```python
from build123d import *

# Parameters (mm, degrees)
F1_DEPTH = 40.2336
F0_R     = 10.16
F2_DEPTH = 15.7734
F3_R     = 3.302


with BuildPart() as f1:
    # F0 (on Front) → F1 (new body)
    with BuildSketch(Plane.XZ):
        with BuildLine():
            ThreePointArc((5.543906, -28.032048), (22.07881, -18.139922), (28.575, 0))
            ThreePointArc((28.575, 0), (22.07881, 18.139922), (5.543906, 28.032048))
            ThreePointArc((5.543906, 28.032048), (-28.575, 0), (5.543906, -28.032048))
        make_face()
        with BuildLine():
            ThreePointArc((13.447765, -4.826), (-14.2875, 0), (13.447765, 4.826))
            Line((13.447765, 4.826), (18.5293, 4.826))
            Line((18.5293, 4.826), (18.5293, -4.826))
            Line((18.5293, -4.826), (13.447765, -4.826))
        make_face(mode=Mode.SUBTRACT)
    extrude(amount=F1_DEPTH)

    # F0 (on Front) → F2 (join)
    with BuildSketch(Plane.XZ):
        with BuildLine():
            ThreePointArc((5.543906, 28.032048), (22.07881, 18.139922), (28.575, 0))
            ThreePointArc((28.575, 0), (22.07881, -18.139922), (5.543906, -28.032048))
            Line((5.543906, -28.032048), (59.169933, -18.327989))
            ThreePointArc((59.169933, -18.327989), (69.171479, -11.487798), (73.025, 0))
            ThreePointArc((73.025, 0), (69.171479, 11.487798), (59.169933, 18.327989))
            Line((59.169933, 18.327989), (5.543906, 28.032048))
        make_face()
        with Locations((53.975, 0)):
            Circle(F0_R, mode=Mode.SUBTRACT)
    extrude(amount=F2_DEPTH)

    # F3
    f3_edges = [f1.edges().sort_by_distance(p)[0] for p in [
        (-5.543906, -40.2336, 28.032048),
    ]]
    fillet(f3_edges, radius=F3_R)


solid = f1.part
```
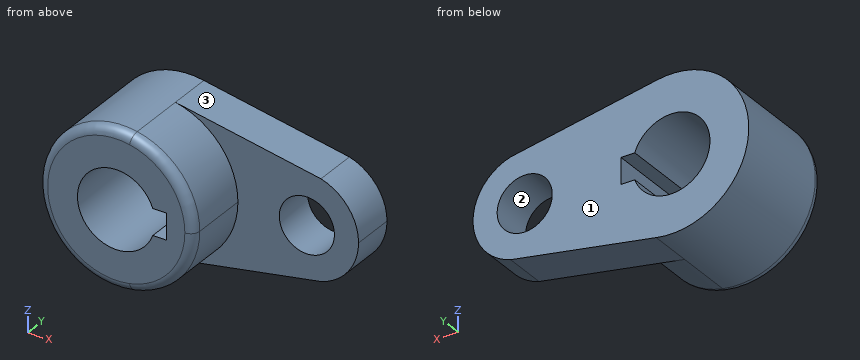
Source: CAD feature listing. Evaluate the final solid. Frame: model axes, mm. Face numbers are marked on the shaded views. Coordinates: 2 decimals unless noted, no trailing zeros. Put each result on its own line as item: value. Start each with the question number.
1) Pull-direction query (Z, two-part tool) for the marked faces 1, 2 and 3; classes: pulls with the +Z half, pulls with the -Z half, needs draft (parallel to the pull), parting line crosses it, or undercut.
2) Ray query, L1, parallel to X at y = -18.5, z = 0 (1 decimal); L2, parallel to Z at x = 0, y = -15 (1 decimal); L3, parallel to X at y = -7, z = -8.5. Return the intervals inside material, ascending. Write a range as from..to.
3) Contact query for flat-ended pins moving along their axis: pin 1 Ø5.5 at (x, y) = (17, -13) entering from -Z; pin 2 Ø4 at (x, y) = (16, -16.5) entering from +Z; pin 3 Ø8 at (x, z) = (36.5, -10.5) entering from -Y. Output: stop coordinate, or through.
4) Cut plane A-A on y = -5. Give the number of separate pieces and of enclosed holes in the cut face, then the cut area to 3 significant figures.
The answers:
1. face 1: needs draft
1. face 2: undercut
1. face 3: pulls with the +Z half
2. L1: x = -28.6..-14.3, 18.5..28.6
2. L2: z = -28.6..-14.3, 14.3..28.6
2. L3: x = -27.28..-11.48, 11.48..48.41, 59.54..71.02
3. pin 1: stops at z = -26.46
3. pin 2: stops at z = 26.48
3. pin 3: stops at y = -15.77
4. separate pieces: 1
4. enclosed holes: 2
4. area: 3,450 mm²
